Verification items for the finished model (mm, model axes). A direction names the side the tool comes from. Round coordinates to 2 decimals unless told otherwise and drop trailing zeros. Write each loop counter-clockwise with the first axis right and the second up, starting at its lowest first coordinate (ties: lowest second). Pieces come first, ordered by that corner, then holes. Notation, with made-up numbers: (8, -20.75) - (67, -20.75) arc R22 ccw to (67, -0.75) - close; hole circle Ø6 at (-38.5, 43.25). An arc over 180 degrees is marked (long way). Answer as a JSON object with one key per item and string values. Group by question number.
1) Section check D-D (y = -2.5). Enter the section's corners in (x, z).
2) Thickness scan on line 1 (X direction, y = -3.25, z = 2.5); line 2 (Z direction, x = 30.5, y = -6.5); line 3 (Y direction, x = 31, z = 1.25). Record the ranges inside material, lowest first.
3) Section check B-B (x = 19.5). Enter the section's corners in (y, z).
4) Go/stop test with flat-tipped pins: pin 1 Ø2 at (x, y) = (-31.5, -1.5) entering from +Z; pin 2 Ø1 at (y, z) = (1, 2) entering from +X; pin 3 Ø3 at (y, z) = (-3.5, 2.5) entering from +X. Record where each tip stops, or that it passes through.
5) Set-up check for faces 1 (the flat face through (24, -4.572, 2)), 2 (the flat face through (31.75, -2, 2)), 3 (the flat face through (-31, 5.55, 2)): record each of +Z, -Z, +X, -X, +Y, -Y from which the full face is reachable in a straight line by a thin tool's end or side.
6) Mould release check, pull along X, two halves, no side actions. Record for faces 4 (the flat face through (24, -0.102, 2)), 5 (the flat face through (39.334, -3.735, -1.559)), 6 (the flat face through (-1, 0, 0)), 7 (the flat face through (15.494, -2, 2)): +X half, -X half, draft (parallel to the pull), parting line (faces both ways), or undercut.
7) Section check A-A (z = 1). Enter the section's corners in (x, y).
8) Section check C-C (y = 1.5). Enter the section's corners in (x, z).
```python
from build123d import *

# Parameters (mm, degrees)
F0_W     = 4.318
F0_H     = 11.0998
F0_W_2   = 16.256
F0_H_2   = 4.4704
F1_DEPTH = 3.1623
F2_DEPTH = 3.4798
F3_DEPTH = 3.4036


with BuildPart() as f1:
    # F0 (on Top) → F1 (new body)
    with BuildSketch(Plane.XY):
        Polygon((36.83, 7.366), (-36.83, 7.366), (-41.91, 0), (-36.83, -7.366), (36.83, -7.366), (41.91, 0), align=None)
        with Locations((-31.115, 0)):
            Rectangle(F0_W, F0_H, mode=Mode.SUBTRACT)
        with Locations((23.622, -2.3368)):
            Rectangle(F0_W_2, F0_H_2, mode=Mode.SUBTRACT)
        with Locations((-31.115, 0)):
            Rectangle(F0_W, F0_H)
        with Locations((23.622, -2.3368)):
            Rectangle(F0_W_2, F0_H_2)
    extrude(amount=-F1_DEPTH)

    # F0 (on Top) → F2 (join)
    with BuildSketch(Plane.XY):
        with Locations((23.622, -2.3368)):
            Rectangle(F0_W_2, F0_H_2)
    extrude(amount=F2_DEPTH)

    # F0 (on Top) → F3 (join)
    with BuildSketch(Plane.XY):
        with Locations((-31.115, 0)):
            Rectangle(F0_W, F0_H)
    extrude(amount=F3_DEPTH)


solid = f1.part
```
Returned:
{
 "1": {"outline": "(-40.19, -3.16) - (40.19, -3.16) - (40.19, 0) - (31.75, 0) - (31.75, 3.48) - (15.49, 3.48) - (15.49, 0) - (-28.96, 0) - (-28.96, 3.4) - (-33.27, 3.4) - (-33.27, 0) - (-40.19, 0) - close"},
 "2": {"line 1": "-33.27 to -28.96, 15.49 to 31.75", "line 2": "-3.16 to 0", "line 3": "-4.57 to -0.1"},
 "3": {"outline": "(-7.37, -3.16) - (7.37, -3.16) - (7.37, 0) - (-0.1, 0) - (-0.1, 3.48) - (-4.57, 3.48) - (-4.57, 0) - (-7.37, 0) - close"},
 "4": {"pin 1": "z = 3.4", "pin 2": "x = -28.96", "pin 3": "x = 31.75"},
 "5": {"face 1": "+Z, +X, -Y", "face 2": "+Z, +X, +Y, -Y", "face 3": "+Z, +X, -X, +Y"},
 "6": {"face 4": "draft", "face 5": "+X half", "face 6": "undercut", "face 7": "undercut"},
 "7": {"outline": "(-33.27, -5.55) - (-28.96, -5.55) - (-28.96, 5.55) - (-33.27, 5.55) - close; (15.49, -4.57) - (31.75, -4.57) - (31.75, -0.1) - (15.49, -0.1) - close"},
 "8": {"outline": "(-40.88, -3.16) - (40.88, -3.16) - (40.88, 0) - (-28.96, 0) - (-28.96, 3.4) - (-33.27, 3.4) - (-33.27, 0) - (-40.88, 0) - close"}
}
